Read the model definition and answer for the solid it produces. Units are mm, in the model's axes. A direction names the side the tool comes from. Round coordinates to 2 decimals unless told otherwise and drop trailing zeros. Order: outer loops, then holes, each group sorted by start corner. A loop starts at its lowest first (then second) coordinate and runs counter-clockwise, first axis right, second up. Notation, with made-up numbers: (3.25, -9.5) - (12.25, -9.5) arc R10 cw to (12.25, -5.5) - close; hole circle Ø4 at (56, -34.5). An arc over 180 degrees is marked (long way). Put each result on its own line as item: value. Start each with the question number.
Q1. Which of the six approach directions +Z, -Z, +X, -X, +Y, -Y give full straight-line access (tool end or side, diameter ignored) to faces 4 (the face through (0, 0, 2)), 5 (the face through (-5.29, -11.96, 1.15)), 6 (the face through (13.01, -0.57, 4.63))?
Q2. Section A-A on x = 0 is taken. Give the vertices of the cut face in (y, z), then the cut area to 3 significant figures.
Q3. For a pull along X with two mould halves and no side action, classify faces 1 (the face through (12.5, 0, 4)), 2 (the face through (-7.72, 10.56, 1.15)), 3 (the face through (13, -1.583, 3)) as pulls with the +X half, pulls with the -X half, needs draft (parallel to the pull), parting line crosses it, or undercut.
Q4. Section C-C on y = -5 is taken. Give the vertices of the cut face in (x, z).
Q5. Each of these flat-tipped pins is pushed along its axis until it touches: pin 1 Ø2 at (y, z) = (1, 3.5) entering from +X; pin 2 Ø4 at (x, y) = (7.5, -1.5) entering from +Z; pin 3 Ø1.8 at (x, y) = (3, 0) entering from -Z. Where does it stop, or does it pass through?
Q6. Section B-B on x = 3 is taken. Give the vertices of the cut face in (y, z).
Q7. Section D-D on z = 4.5 is taken. Give the vertices of the cut face in (x, y).
Q8. Find the intervals of material crossed by line 1 along Y through (x, z) = (0, 5.1); line 2 along X through (y, z) = (10, 3.5); line 3 along Z through (x, y) = (4.5, 7), in increasing order. Write a range as from..to.
from build123d import *

# Parameters (mm, degrees)
SKETCH1_R                   = 13.5
BOSS_EXTRUDE1_DEPTH         = 2
SKETCH2_R                   = 13.5
SKETCH2_R_2                 = 12
BOSS_EXTRUDE2_DEPTH         = 4
SKETCH4_R                   = 1
CUT_EXTRUDE1_DEPTH          = 13
SKETCH4_3_R                 = 1
CUT_EXTRUDE2_DEPTH          = 7.5
CIRPATTERN1_COUNT           = 3
CIRPATTERN2_COUNT           = 3
CIRPATTERN2_COPY_1_SKETCH_R = 1
CIRPATTERN2_COPY_1_DEPTH    = 7.5
CIRPATTERN2_COPY_2_SKETCH_R = 1
CIRPATTERN2_COPY_2_DEPTH    = 7.5
CIRPATTERN2_COPY_3_SKETCH_R = 1
CIRPATTERN2_COPY_3_DEPTH    = 7.5
CIRPATTERN2_COPY_4_SKETCH_R = 1
CIRPATTERN2_COPY_4_DEPTH    = 7.5
CIRPATTERN2_COPY_5_SKETCH_R = 1
CIRPATTERN2_COPY_5_DEPTH    = 7.5
CIRPATTERN2_COPY_6_SKETCH_R = 1
CIRPATTERN2_COPY_6_DEPTH    = 7.5
SKETCH5_R                   = 1
CUT_EXTRUDE3_DEPTH          = 20.506409224


with BuildPart() as part:
    # Sketch1 → Boss-Extrude1 (new body)
    with BuildSketch(Plane.XY):
        Circle(SKETCH1_R)
    extrude(amount=BOSS_EXTRUDE1_DEPTH)

    # Sketch2 → Boss-Extrude2 (add)
    with BuildSketch(Plane.XY.offset(2)):
        Circle(SKETCH2_R)
        Circle(SKETCH2_R_2, mode=Mode.SUBTRACT)
    extrude(amount=BOSS_EXTRUDE2_DEPTH)

    # Sketch4 → Cut-Extrude1 (cut)
    with BuildSketch(Plane(origin=(20, 0, 0), x_dir=(0, 0, -1), z_dir=(1, 0, 0))):
        with Locations((-2.890598923, 0.416590766)):
            Circle(SKETCH4_R)
    cut_extrude1 = extrude(amount=-CUT_EXTRUDE1_DEPTH, mode=Mode.SUBTRACT)

    # Sketch4_3 → Cut-Extrude2 (cut)
    with BuildSketch(Plane(origin=(20, 0, 0), x_dir=(0, 0, -1), z_dir=(1, 0, 0))):
        Polygon((-0.581197846, 0.416590766), (-1.735898385, 2.416590766), (-4.045299462, 2.416590766), (-5.2, 0.416590766), (-4.045299462, -1.583409234), (-1.735898385, -1.583409234), align=None)
        with Locations((-2.890598923, 0.416590766)):
            Circle(SKETCH4_3_R, mode=Mode.SUBTRACT)
    cut_extrude2 = extrude(amount=-CUT_EXTRUDE2_DEPTH, mode=Mode.SUBTRACT)

    # CirPattern1: Cut-Extrude2 ×3 about axis
    cirpattern1_axis = Axis((0, 0, 0), (0, 0, 1))
    for i in range(1, CIRPATTERN1_COUNT):
        add(cut_extrude2.rotate(cirpattern1_axis, i * 360 / CIRPATTERN1_COUNT), mode=Mode.SUBTRACT)

    # CirPattern2: Cut-Extrude1 ×3 about axis
    cirpattern2_axis = Axis((0, 0, 0), (0, 0, 1))
    for i in range(1, CIRPATTERN2_COUNT):
        add(cut_extrude1.rotate(cirpattern2_axis, i * 360 / CIRPATTERN2_COUNT), mode=Mode.SUBTRACT)

    # CirPattern2 copy 1 sketch → CirPattern2 copy 1 (cut)
    with BuildSketch(Plane(origin=(-10, -17.320508076, 0), x_dir=(0, 0, -1), z_dir=(-0.5000000000000003, -0.8660254037844384, 0))):
        Polygon((-0.581197846, 0.416590766), (-1.735898385, 2.416590766), (-4.045299462, 2.416590766), (-5.2, 0.416590766), (-4.045299462, -1.583409234), (-1.735898385, -1.583409234), align=None)
        with Locations((-2.890598923, 0.416590766)):
            Circle(CIRPATTERN2_COPY_1_SKETCH_R, mode=Mode.SUBTRACT)
    extrude(amount=-CIRPATTERN2_COPY_1_DEPTH, mode=Mode.SUBTRACT)

    # CirPattern2 copy 2 sketch → CirPattern2 copy 2 (cut)
    with BuildSketch(Plane(origin=(20, 0, 0), x_dir=(0, 0, -1), z_dir=(1, 0, 0))):
        Polygon((-0.581197846, 0.416590766), (-1.735898385, 2.416590766), (-4.045299462, 2.416590766), (-5.2, 0.416590766), (-4.045299462, -1.583409234), (-1.735898385, -1.583409234), align=None)
        with Locations((-2.890598923, 0.416590766)):
            Circle(CIRPATTERN2_COPY_2_SKETCH_R, mode=Mode.SUBTRACT)
    extrude(amount=-CIRPATTERN2_COPY_2_DEPTH, mode=Mode.SUBTRACT)

    # CirPattern2 copy 3 sketch → CirPattern2 copy 3 (cut)
    with BuildSketch(Plane(origin=(20, 0, 0), x_dir=(0, 0, -1), z_dir=(1, 0, 0))):
        Polygon((-0.581197846, 0.416590766), (-1.735898385, 2.416590766), (-4.045299462, 2.416590766), (-5.2, 0.416590766), (-4.045299462, -1.583409234), (-1.735898385, -1.583409234), align=None)
        with Locations((-2.890598923, 0.416590766)):
            Circle(CIRPATTERN2_COPY_3_SKETCH_R, mode=Mode.SUBTRACT)
    extrude(amount=-CIRPATTERN2_COPY_3_DEPTH, mode=Mode.SUBTRACT)

    # CirPattern2 copy 4 sketch → CirPattern2 copy 4 (cut)
    with BuildSketch(Plane(origin=(-10, 17.320508076, 0), x_dir=(0, 0, -1), z_dir=(-0.4999999999999991, 0.8660254037844392, 0))):
        Polygon((-0.581197846, 0.416590766), (-1.735898385, 2.416590766), (-4.045299462, 2.416590766), (-5.2, 0.416590766), (-4.045299462, -1.583409234), (-1.735898385, -1.583409234), align=None)
        with Locations((-2.890598923, 0.416590766)):
            Circle(CIRPATTERN2_COPY_4_SKETCH_R, mode=Mode.SUBTRACT)
    extrude(amount=-CIRPATTERN2_COPY_4_DEPTH, mode=Mode.SUBTRACT)

    # CirPattern2 copy 5 sketch → CirPattern2 copy 5 (cut)
    with BuildSketch(Plane(origin=(-10, 17.320508076, 0), x_dir=(0, 0, -1), z_dir=(-0.4999999999999998, 0.8660254037844387, 0))):
        Polygon((-0.581197846, 0.416590766), (-1.735898385, 2.416590766), (-4.045299462, 2.416590766), (-5.2, 0.416590766), (-4.045299462, -1.583409234), (-1.735898385, -1.583409234), align=None)
        with Locations((-2.890598923, 0.416590766)):
            Circle(CIRPATTERN2_COPY_5_SKETCH_R, mode=Mode.SUBTRACT)
    extrude(amount=-CIRPATTERN2_COPY_5_DEPTH, mode=Mode.SUBTRACT)

    # CirPattern2 copy 6 sketch → CirPattern2 copy 6 (cut)
    with BuildSketch(Plane(origin=(-10, -17.320508076, 0), x_dir=(0, 0, -1), z_dir=(-0.5000000000000004, -0.8660254037844384, 0))):
        Polygon((-0.581197846, 0.416590766), (-1.735898385, 2.416590766), (-4.045299462, 2.416590766), (-5.2, 0.416590766), (-4.045299462, -1.583409234), (-1.735898385, -1.583409234), align=None)
        with Locations((-2.890598923, 0.416590766)):
            Circle(CIRPATTERN2_COPY_6_SKETCH_R, mode=Mode.SUBTRACT)
    extrude(amount=-CIRPATTERN2_COPY_6_DEPTH, mode=Mode.SUBTRACT)

    # Sketch5 → Cut-Extrude3 (cut, through all)
    with BuildSketch(Plane.XY.offset(2)):
        with Locations((3, 0)):
            Circle(SKETCH5_R)
        with Locations((-3, 0)):
            Circle(SKETCH5_R)
    extrude(amount=-CUT_EXTRUDE3_DEPTH, mode=Mode.SUBTRACT)


solid = part.part
Findings:
1. face 4: +Z
1. face 5: none
1. face 6: +X
2. outline: (-13.5, 0) - (13.5, 0) - (13.5, 6) - (12, 6) - (12, 2) - (-12, 2) - (-12, 6) - (-13.5, 6) - close
2. area: 66.0 mm2
3. face 1: pulls with the +X half
3. face 2: undercut
3. face 3: needs draft
4. outline: (-12.54, 0) - (12.54, 0) - (12.54, 6) - (10.91, 6) - (10.91, 2) - (-10.91, 2) - (-10.91, 6) - (-12.54, 6) - close
5. pin 1: x = 12.5
5. pin 2: z = 2
5. pin 3: through
6. outline: (-13.16, 0) - (-1, 0) - (-1, 2) - (-11.62, 2) - (-11.62, 6) - (-13.16, 6) - close; (1, 0) - (13.16, 0) - (13.16, 6) - (11.62, 6) - (11.62, 2) - (1, 2) - close
7. outline: (-8.11, 10.79) arc R13.5 ccw to (-7.43, -11.27) - (-6.94, -10.43) - (-4.84, -11.64) - (-5.29, -12.42) arc R13.5 ccw to (13.48, -0.8) - (12.5, -0.8) - (12.5, 1.63) - (13.4, 1.63) arc R13.5 ccw to (-6.05, 12.07) - (-5.56, 11.22) - (-7.66, 10.01) - close; hole circle Ø24 at (0, 0)
8. line 1: -13.5..-12, 12..13.5
8. line 2: -9.07..-8.56, -7.68..-7.17, 6.63..9.07
8. line 3: 0..2
